Read the model definition and answer for the solid it produces. Units are mm, in the model's axes. A direction names the side the tool comes from. Round coordinates to 2 decimals unless told otherwise and drop trailing zeros. Write each loop counter-clockwise with the first axis right and the second up, starting at its lowest first coordinate (ties: lowest second). Pieces come first, ordered by that corner, then holes. Notation, with made-up numbers: (13.25, -23.5) -> (66.25, -23.5) arc R36 cw to (66.25, 11.5) -> close; hole circle Ø5 at (67, 67). An arc over 180 degrees is marked (long way). Return JSON: item names as keys, results as strings.
from build123d import *

# Parameters (mm, degrees)
F0_W     = 50.8
F0_H     = 50.8
F1_DEPTH = 12.7
F2_W     = 38.1
F2_H     = 44.45
F3_DEPTH = 25.4
F5_DEPTH = 47.752


with BuildPart() as f1:
    # F0 (on Top) → F1 (new body)
    with BuildSketch(Plane.XY):
        Rectangle(F0_W, F0_H)
    extrude(amount=F1_DEPTH)

    # F2 (on face) → F3 (cut)
    with BuildSketch(Plane.XY.offset(12.7)):
        with Locations((0, -3.175)):
            Rectangle(F2_W, F2_H)
    extrude(amount=-F3_DEPTH, mode=Mode.SUBTRACT)

    # F4 (on face) → F5 (join)
    with BuildSketch(Plane.YZ.offset(25.4)):
        Polygon((20.342838, 0), (-25.4, 12.7), (-25.4, 0), align=None)
    extrude(amount=-F5_DEPTH)


solid = f1.part
Item 1: For a pull along X with two mould halves and no side action, classify faces 1 (the flat face through (19.05, 6, 9)), 2 (the flat face through (-2, 21, 12.7)), 3 (the flat face through (25.4, 0, 6)) as released by +X, released by -X, zero draft, split by the parting line, or undercut.
Worked answers:
{"face 1": "undercut", "face 2": "zero draft", "face 3": "released by +X"}
Item 2: Section A-A (z = 9.75) is taken. Give the vertices of the cut face in (x, y).
Worked answers:
{"outline": "(-25.4, -25.4) -> (25.4, -25.4) -> (25.4, 25.4) -> (-25.4, 25.4) -> close; hole (-19.05, -14.77) -> (19.05, -14.77) -> (19.05, 19.05) -> (-19.05, 19.05) -> close"}
Item 3: Section C-C (y = -22) is taken. Give the vertices of the cut face in (x, z), then the cut area to 3 significant figures.
Worked answers:
{"outline": "(-25.4, 0) -> (25.4, 0) -> (25.4, 12.7) -> (19.05, 12.7) -> (19.05, 11.76) -> (-19.05, 11.76) -> (-19.05, 12.7) -> (-25.4, 12.7) -> close", "area": "609 mm2"}
Item 4: Section D-D (z = 2.75) is taken. Give the vertices of the cut face in (x, y), then the cut area to 3 significant figures.
Worked answers:
{"outline": "(-25.4, -25.4) -> (25.4, -25.4) -> (25.4, 25.4) -> (-25.4, 25.4) -> close; hole (-19.05, 10.44) -> (19.05, 10.44) -> (19.05, 19.05) -> (-19.05, 19.05) -> close", "area": "2,250 mm2"}
Item 5: Section B-B (x = -9) is taken. Give the vertices of the cut face in (y, z), then the cut area to 3 significant figures.
Worked answers:
{"outline": "(-25.4, 0) -> (25.4, 0) -> (25.4, 12.7) -> (19.05, 12.7) -> (19.05, 0.36) -> (-25.4, 12.7) -> close", "area": "371 mm2"}
Item 6: A tool of negligible diameter and unlimited length cuts with its end or side. For faces 4 (the flat face through (0, 19.05, 7)), 5 (the flat face through (-25.4, 0, 6)), from which of +Z, -Z, +X, -X, +Y, -Y can it reach the whole face along a straight path? Write none if from no direction.
Worked answers:
{"face 4": "+Z", "face 5": "+Z, -Z, -X, +Y, -Y"}
Item 7: Straight lines are drawn through the part: L1, parallel to X at y = -19.5, z = 11.75; L2, parallel to Z at x = 14.5, y = 0.5; L3, parallel to Z at x = -3.5, y = 11.5. For each, find the intervals that lie inside material, in ascending order. Write a range as [from, to].
Worked answers:
{"L1": "x = [-25.4, -19.05], [19.05, 25.4]", "L2": "z = [0, 5.51]", "L3": "z = [0, 2.46]"}
Item 8: A flat-ended cylindrical pin translates along its axis: pin 1 (1 mm diameter, centred on x = 10.5, y = -17.5, fed in from +Z). Find the tip coordinate at first contact, or state that the pin passes through.
Worked answers:
{"pin 1": "stops at z = 10.65"}
